```python
from build123d import *

# Parameters (mm, degrees)
SKETCH1_W           = 208.6
SKETCH1_H           = 80.8
SKETCH1_R           = 4
SKETCH1_W_2         = 20
SKETCH1_H_2         = 30
BOSS_EXTRUDE1_DEPTH = 8
SKETCH1_3_W         = 20
SKETCH1_3_H         = 30
BOSS_EXTRUDE2_DEPTH = 30
FILLET1_R           = 5
FILLET2_R           = 15
SKETCH2_R           = 5
CUT_EXTRUDE1_DEPTH  = 462.279122908


with BuildPart() as part:
    # Sketch1 → Boss-Extrude1 (new body)
    # profile 1 of 3: a face of its own
    with BuildSketch(Plane.XY):
        with Locations((21.844388387, -381.87501611)):
            Rectangle(SKETCH1_W, SKETCH1_H)
        with Locations((113.444388387, -409.57501611)):
            Circle(SKETCH1_R, mode=Mode.SUBTRACT)
        with Locations((-69.755611613, -354.17501611)):
            Circle(SKETCH1_R, mode=Mode.SUBTRACT)
        with Locations((-69.755611613, -409.57501611)):
            Circle(SKETCH1_R, mode=Mode.SUBTRACT)
        with Locations((113.444388387, -354.17501611)):
            Circle(SKETCH1_R, mode=Mode.SUBTRACT)
        with Locations((90.744388387, -381.87501611)):
            Rectangle(SKETCH1_W_2, SKETCH1_H_2, mode=Mode.SUBTRACT)
        with Locations((-47.055611613, -381.87501611)):
            Rectangle(SKETCH1_W_2, SKETCH1_H_2, mode=Mode.SUBTRACT)
    # profile 2 of 3: a face of its own
    with BuildSketch(Plane.XY):
        with Locations((-47.055611613, -381.87501611)):
            Rectangle(SKETCH1_W_2, SKETCH1_H_2)
    # profile 3 of 3: a face of its own
    with BuildSketch(Plane.XY):
        with Locations((90.744388387, -381.87501611)):
            Rectangle(SKETCH1_W_2, SKETCH1_H_2)
    extrude(amount=BOSS_EXTRUDE1_DEPTH)

    # Sketch1<3> → Boss-Extrude2 (add)
    with BuildSketch(Plane.XY):
        with Locations((90.744388387, -381.87501611)):
            Rectangle(SKETCH1_3_W, SKETCH1_3_H)
        with Locations((-47.055611613, -381.87501611)):
            Rectangle(SKETCH1_3_W, SKETCH1_3_H)
    extrude(amount=-BOSS_EXTRUDE2_DEPTH)

    # Fillet1
    fillet1_edges = [part.edges().sort_by_distance(p)[0] for p in [
        (90.744388387, -366.87501611, 0),
        (90.744388387, -396.87501611, 0),
        (-47.055611613, -366.87501611, 0),
        (-47.055611613, -396.87501611, 0),
    ]]
    fillet(fillet1_edges, radius=FILLET1_R)

    # Fillet2
    fillet2_edges = [part.edges().sort_by_distance(p)[0] for p in [
        (90.744388387, -366.87501611, -30),
        (90.744388387, -396.87501611, -30),
        (-47.055611613, -396.87501611, -30),
        (-47.055611613, -366.87501611, -30),
    ]]
    fillet(fillet2_edges, radius=FILLET2_R - 0.0001)  # a hair under: the kernel refuses the full size

    # Sketch2 → Cut-Extrude1 (cut, through all)
    with BuildSketch(Plane(origin=(100.744388387, 0, 0), x_dir=(0, 0, -1), z_dir=(1, 0, 0))):
        with Locations(Location((15, -381.87501611, 0), (0, 0, 90))):
            Circle(SKETCH2_R)
    extrude(amount=-CUT_EXTRUDE1_DEPTH, mode=Mode.SUBTRACT)


solid = part.part
```
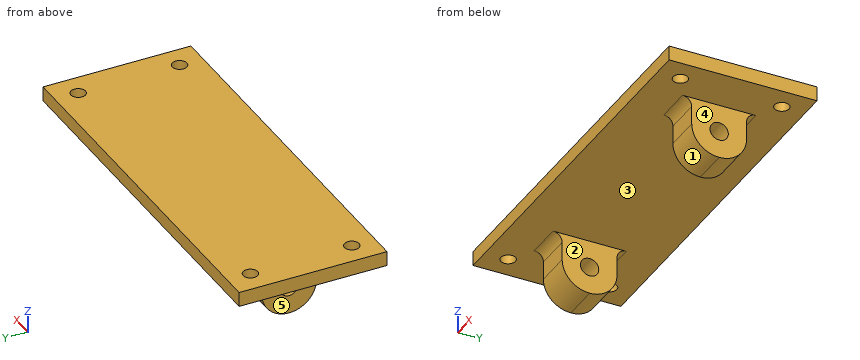
The listing builds one solid part. Answer for the finished solid, in the listing's coordinates (mm). Face numbers are marked on the shaded views. A direction names the side the tool comes from. Coordinates: 2 decimals unless noted, no trailing zeros. Write each loop counter-clockwise with the first axis right and the second up, starting at its lowest first coordinate (ties: lowest second). Pieces come first, ordered by that corner, then holes. Notation, with made-up numbers: (87, -7) - (112, -7) arc R22 ccw to (112, 30) - close; hole circle Ø4 at (-26, 29). An arc over 180 degrees is marked (long way). Return JSON: item names as keys, results as strings. Group by question number.
1. Which of the six approach directions +Z, -Z, +X, -X, +Y, -Y give full straight-line access (tool end or side, diameter ignored) to the marked faces 1 and 2?
2. A cutting plane is placed at C-C, the plane x = -17. Determine the outline of the cut face in (y, z).
3. Given pin 1 (6 mm diameter, centred on x = 53, y = -386.5, fed in from -Z); pin 2 (11 mm diameter, centred on x = -50.5, z = -10, fed in from -Y); pin 3 (3 mm diameter, centred on x = -50, z = -10, fed in from +Y) (3 decimals), each flat-ended and moving along its own axis, determine where each tip first touches the part or whether it passes through.
4. Straight lines are drawn through the part: L1, parallel to X at y = -410, z = 4; L2, parallel to X at y = -373, z = -6.5; L3, parallel to Z at x = 76, y = -376.5. For each, find the intervals that lie inside material, in ascending order.
5. Determine the mould class of the marked faces 3, 4 and 5 for opening direction X: released by +X, released by -X, zero draft, split by the parting line, or undercut.
6. A cutting plane is placed at A-A, the plane z = -18. Determine the outline of the cut face in (x, y), plus the area to 3 significant figures.
Ans:
{
 "1": {"face 1": "-Z, +X, -X, -Y", "face 2": "-Z, +Y, -Y"},
 "2": {"outline": "(-422.28, 0) - (-341.48, 0) - (-341.48, 8) - (-422.28, 8) - close"},
 "3": {"pin 1": "z = 0", "pin 2": "y = -396.9", "pin 3": "y = -366.875"},
 "4": {"L1": "-82.46 to -73.73, -65.78 to 109.47, 117.42 to 126.14", "L2": "-57.06 to -37.06, 80.74 to 100.74", "L3": "0 to 8"},
 "5": {"face 3": "undercut", "face 4": "released by +X", "face 5": "released by -X"},
 "6": {"outline": "(-57.06, -396.57) - (-37.06, -396.57) - (-37.06, -385.88) - (-57.06, -385.88) - close; (-57.06, -377.88) - (-37.06, -377.88) - (-37.06, -367.18) - (-57.06, -367.18) - close; (80.74, -396.57) - (100.74, -396.57) - (100.74, -385.88) - (80.74, -385.88) - close; (80.74, -377.88) - (100.74, -377.88) - (100.74, -367.18) - (80.74, -367.18) - close", "area": "856 mm²"}
}
